Autodesk Inventor part; units mm, degrees
ref_plane "YZ Plane" through (0, 0, 0) normal (1, 0, 0) x (0, 1, 0)
ref_plane "XZ Plane" through (0, 0, 0) normal (0, 1, 0) x (-1, 0, 0)
ref_plane "XY Plane" through (0, 0, 0) normal (0, 0, 1) x (1, 0, 0)
sketch "Sketch1" plane through (0, 0, 0) normal (0, 0, 1) x (1, 0, 0)
  line L0 (-12.7, -19.05) -> (12.7, -19.05)
  line L1 (12.7, -19.05) -> (12.7, 19.05)
  line L2 (12.7, 19.05) -> (-12.7, 19.05)
  line L3 (-12.7, 19.05) -> (-12.7, -19.05)
  line L4 (-12.7, -19.05) -> (12.7, 19.05) construction
  line L5 (12.7, -19.05) -> (-12.7, 19.05) construction
  line L6 (-9.525, 15.875) -> (9.525, 15.875)
  line L7 (9.525, 15.875) -> (9.525, -15.875)
  line L8 (9.525, -15.875) -> (-9.525, -15.875)
  line L9 (-9.525, -15.875) -> (-9.525, 15.875)
  point P0 (0, 0)
  dimension "d0" = 25.4
  dimension "d1" = 38.1
  dimension "d2" = 3.175
extrude "Extrusion1" add sketch "Sketch1" along normal mid plane 127
sketch "Sketch2" plane through (12.7, -19.05, 63.5) normal (1, 0, 0) x (0, 0, -1)
  circle A0 centre (63.5, 19.05) radius 3.175
  dimension "d5" = 6.35
extrude "Extrusion2" cut sketch "Sketch2" against normal through all
pattern_linear "Rectangular Pattern1" count 4 spacing 25.4 along (0, 0, 1) of "Extrusion2" first direction both ways yes
hole "Hole1" at (12.7, 0, 0) direction (-1, 0, 0) diameter 15.875 end through all
hole "Hole2" at (12.7, 0, 0) direction (-1, 0, 0) diameter 19.05 end through all
sketch "Sketch3" plane through (12.7, -19.05, 63.5) normal (1, 0, 0) x (0, 0, -1)
  line L0 (127, 38.1) -> (0, 38.1)
  line L1 (63.5, 38.1) -> (63.5, 0)
  line L2 (0, 0) -> (127, 0)
  line L3 (25.4, 38.1) -> (25.4, 0)
  line L4 (0, 0) -> (0, 38.1)
  line L5 (101.6, 38.1) -> (101.6, 0)
  line L6 (127, 38.1) -> (127, 0)
  point P0 (63.5, 19.05)
  dimension "d29" = 25.4
  dimension "d30" = 25.4
split body "Split1" sketch "Sketch3" result one side removed curves L3 removed pieces at (12.2, -13.7506, 50.6724)
split body "Split2" sketch "Sketch3" result one side removed curves L5 removed pieces at (12.2, -6.35, -55.0333)
properties part number "2AM-17-P-5209 - cylinder mount" material "Aluminum 6061"
Work out the finished part from the listing and answer in its coordinate system (mm). A direction names the side the tool comes from. Round coordinates to 2 decimals unless told otherwise and drop trailing zeros. Write each loop counter-clockwise with the first axis right and the second up, starting at its lowest first coordinate (ties: lowest second). Pieces come first, ordered by that corner, then holes. Notation, with made-up numbers: (34, -33.5) -> (78, -33.5) arc R20 cw to (78, -20.5) -> close; hole circle Ø10 at (-15.75, -29). An arc over 180 degrees is marked (long way). Write each question's results on one line, items separated by ' | '.
Q1. Section B-B, the plane y = 12.5 is taken. Write down the section's boundary in (x, z) (3 decimals), then the cut area to 3 significant figures.
Data:
outline: (-12.7, -38.1) -> (-9.525, -38.1) -> (-9.525, 38.1) -> (-12.7, 38.1) -> close; (9.525, -38.1) -> (12.7, -38.1) -> (12.7, 38.1) -> (9.525, 38.1) -> close | area: 484 mm^2
Q2. Section C-C, the plane x = -10.75 is taken. Write down the section's boundary in (y, z) (3 decimals), then the cut area to 3 significant figures.
Data:
outline: (-19.05, -38.1) -> (19.05, -38.1) -> (19.05, 38.1) -> (-19.05, 38.1) -> close; hole circle Ø19.05 at (0, 0); hole circle Ø6.35 at (0, -25.4); hole circle Ø6.35 at (0, 25.4) | area: 2,550 mm^2
Q3. Determine the mould class of faces 3 (the flat face through (-11, 0, 38.1)), 4 (the flat face through (0, 15.875, -1)), 5 (the flat face through (11, 0, -38.1)), 6 (the cylindrical face through (-11.09, 0.95, 22.37)) for opening direction Z: released by +Z, released by -Z, zero draft, split by the parting line, or undercut.
Data:
face 3: released by +Z | face 4: zero draft | face 5: released by -Z | face 6: undercut
Q4. Straight lines are drawn through the part: line 1 along X through (y, z) = (14, 9.5) (3 decimals); line 2 along Y through (x, z) = (-11.85, 25.4) (3 decimals); line 3 along Y through (x, z) = (11.35, 0) (3 decimals). For each, find the intervals that lie inside material, in ascending order. Write a range as [from, to].
Data:
line 1: [-12.7, -9.525], [9.525, 12.7] | line 2: [-19.05, -3.175], [3.175, 19.05] | line 3: [-19.05, -9.525], [9.525, 19.05]
Q5. Section A-A, the plane z = -25.4 is taken. Write down the section's boundary in (x, y) (3 decimals).
Data:
outline: (-12.7, -19.05) -> (12.7, -19.05) -> (12.7, -3.175) -> (9.525, -3.175) -> (9.525, -15.875) -> (-9.525, -15.875) -> (-9.525, -3.175) -> (-12.7, -3.175) -> close; (-12.7, 3.175) -> (-9.525, 3.175) -> (-9.525, 15.875) -> (9.525, 15.875) -> (9.525, 3.175) -> (12.7, 3.175) -> (12.7, 19.05) -> (-12.7, 19.05) -> close
Q6. Which of the six approach directions +Z, -Z, +X, -X, +Y, -Y give full straight-line access (tool end or side, diameter ignored) to faces 1 (the flat face through (9.525, 4, -9)), 2 (the flat face through (12.7, 4, -9))?
Data:
face 1: +Z, -Z | face 2: +Z, -Z, +X, +Y, -Y
Q7. Section D-D, the plane y = 0 is taken. Give the number of separate pieces and of enclosed holes in the cut face, then the cut area to 3 significant figures.
Data:
separate pieces: 8 | enclosed holes: 0 | area: 282 mm^2
